Verification items for this drawing (mm, ordinates from the low corner). A direction names the side the tool comes from. Give positions to 0.01 mm unless a question says otherwise; leave off trailing zeros. Loops run counter-clockwise (first coordinate to the right, second up) from the corner with the lowest first, then second, coordinate; pieces in that order, holes last. Notation, with made-up numbers: (54.25, 13) - (109.25, 13) arc R7 ccw to (109.25, 26) - close; hole circle Ø2 at (59.25, 60.25). An arc over 180 degrees is marked (long way). Write item = value, one per line. Start each with the question number.
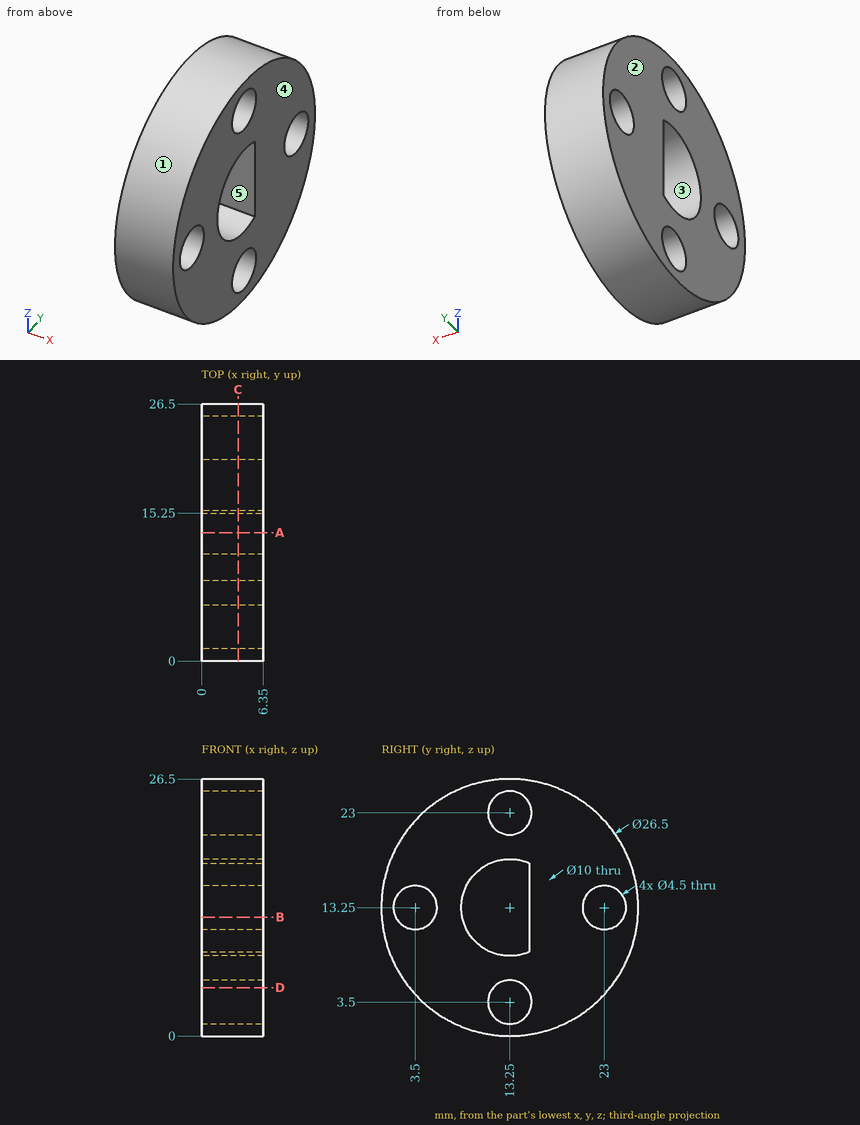
1) Gauge pin test, flat ends, axial feed: P1, Ø1.5, axis at x = 4.5, z = 20, coming from the -Y side; P2, Ø2.5, axis at y = 13.25, z = 23, coming from the -X side; P3, Ø2, axis at x = 2, z = 21.5, coming from the +Y side; P4, Ø1.9, axis at x = 4, z = 11.5, coming from the -Y side. Record the tip position at first contact, or that the pin passes through.
2) Cross-section at C-C on x = 3.75. Enter the section's corners in (y, z), and give its area (3 significant figures).
3) Material ranges on line 1 along Y through (x, z) = (3.5, 13.25); line 2 along Y through (x, z) = (2.75, 14.5); line 3 along Z through (x, y) = (2.25, 10.5), recorded low to high.
4) Release check for a two-part mould opening along Y. For the marked faces 1, 2 and 3 record: pulls with the +Y half, pulls with the -Y half, needs draft (parallel to the pull), parting line crosses it, or undercut.
5) Tool access check on the marked faces 4 and 5. Record the directions out of +Z, -Z, +X, -X, +Y, -Y that give a thin tool (end or side, any length) a straight path to the whole face; none if there is none.
6) Cross-section at B-B on z = 12.25. Enter the section's corners in (x, y), and give its area (3 significant figures).
7) Cross-section at D-D on z = 5. Enter the section's corners in (x, y), and give its area (3 significant figures).
8) Cross-section at A-A on y = 13.25. Enter the section's corners in (x, z).
Checked values:
q1.P1 = 1.44
q1.P2 = through
q1.P3 = 24.34
q1.P4 = 0.02
q2.outline = circle Ø26.5 at (13.25, 13.25); hole circle Ø4.5 at (3.5, 13.25); hole circle Ø4.5 at (13.25, 3.5); hole circle Ø4.5 at (13.25, 23); hole (15.25, 8.67) - (15.25, 17.83) arc R5 ccw (long way) to start; hole circle Ø4.5 at (23, 13.25)
q2.area = 429 mm²
q3.line_1 = 0 to 1.25, 5.75 to 8.25, 15.25 to 20.75, 25.25 to 26.5
q3.line_2 = 0.06 to 1.63, 5.37 to 8.41, 15.25 to 21.13, 24.87 to 26.44
q3.line_3 = 0.29 to 9.07, 17.43 to 26.21
q4.face_1 = parting line crosses it
q4.face_2 = needs draft
q4.face_3 = undercut
q5.face_4 = +Z, -Z, +X, +Y, -Y
q5.face_5 = +X, -X
q6.outline = (0, 0.04) - (6.35, 0.04) - (6.35, 1.48) - (0, 1.48) - close; (0, 5.52) - (6.35, 5.52) - (6.35, 8.35) - (0, 8.35) - close; (0, 15.25) - (6.35, 15.25) - (6.35, 20.98) - (0, 20.98) - close; (0, 25.02) - (6.35, 25.02) - (6.35, 26.46) - (0, 26.46) - close
q6.area = 72.8 mm²
q7.outline = (0, 2.88) - (6.35, 2.88) - (6.35, 11.57) - (0, 11.57) - close; (0, 14.93) - (6.35, 14.93) - (6.35, 23.62) - (0, 23.62) - close
q7.area = 110 mm²
q8.outline = (0, 0) - (6.35, 0) - (6.35, 1.25) - (0, 1.25) - close; (0, 5.75) - (6.35, 5.75) - (6.35, 8.25) - (0, 8.25) - close; (0, 18.25) - (6.35, 18.25) - (6.35, 20.75) - (0, 20.75) - close; (0, 25.25) - (6.35, 25.25) - (6.35, 26.5) - (0, 26.5) - close
